```python
from build123d import *
from build123d.topology import SkipClean

# Parameters (mm, degrees)
EXTRUDE_1_DEPTH          = 2.75
SKETCH_2_R               = 9.5
CUT_EXTRUDE_1_DEPTH      = 87.748932825
SKETCH_3_R               = 1.65
CUT_EXTRUDE_2_DEPTH      = 87.748932825
CUT_EXTRUDE_3_DEPTH      = 87.748932825
CUT_EXTRUDE_3_DEPTH_BACK = 87.748932825
SKETCH_4_R               = 13
PATTERN_CIRCULAR_1_COUNT = 4
SKETCH_6_R               = 1.6
CUT_EXTRUDE_5_DEPTH      = 87.748932825
CUT_EXTRUDE_4_DEPTH      = 87.748932825
CUT_EXTRUDE_4_DEPTH_BACK = 87.748932825
SKETCH_5_R               = 15
CUT_EXTRUDE_7_DEPTH      = 87.748932825
CUT_EXTRUDE_7_DEPTH_BACK = 87.748932825
SKETCH_8_R               = 1.6


with BuildPart() as part:
    # ｽｹｯﾁ1 → ﾎﾞｽ - 押し出し1 (new, symmetric)
    with BuildSketch(Plane.XY):
        with BuildLine():
            Line((17.5, 0), (-47.316776584, 0))
            Line((-47.316776584, 0), (-47.316776584, -50))
            ThreePointArc((-47.316776584, -50), (-28.966828956, -72.113956347), (-3.847704112, -58.157695734))
            Line((-3.847704112, -58.157695734), (16.309278589, -6.34487446))
            ThreePointArc((16.309278589, -6.34487446), (17.199743825, -3.227818512), (17.5, 0))
        make_face()
    extrude_1 = extrude(amount=EXTRUDE_1_DEPTH, both=True)

    # ｽｹｯﾁ2 → ｶｯﾄ - 押し出し1 (cut, symmetric)
    with BuildSketch(Plane.XY.offset(2.75)):
        Circle(SKETCH_2_R)
    cut_extrude_1 = extrude(amount=CUT_EXTRUDE_1_DEPTH, both=True, mode=Mode.SUBTRACT)

    # ｽｹｯﾁ3 → ｶｯﾄ - 押し出し2 (cut, symmetric)
    with BuildSketch(Plane.XY.offset(2.75)):
        with Locations((-24.816776584, -67.5)):
            Circle(SKETCH_3_R)
    cut_extrude_2 = extrude(amount=CUT_EXTRUDE_2_DEPTH, both=True, mode=Mode.SUBTRACT)

    # ｽｹｯﾁ4 → ｶｯﾄ - 押し出し3 (cut, two sides: drawn at the far end of the back side and taken through both)
    with BuildSketch(Plane.XY.offset(2.75).offset(-CUT_EXTRUDE_3_DEPTH_BACK)):
        with Locations((-24.816776584, -50)):
            Circle(SKETCH_4_R)
    extrude(amount=CUT_EXTRUDE_3_DEPTH + CUT_EXTRUDE_3_DEPTH_BACK, mode=Mode.SUBTRACT)

    # 円形ﾊﾟﾀｰﾝ1: ｶｯﾄ - 押し出し2 ×4 about axis
    pattern_circular_1_axis = Axis((-24.816776584, -50, 0), (0, 0, 1))
    for i in range(1, PATTERN_CIRCULAR_1_COUNT):
        add(cut_extrude_2.rotate(pattern_circular_1_axis, i * 360 / PATTERN_CIRCULAR_1_COUNT), mode=Mode.SUBTRACT)

    # ｽｹｯﾁ6 → ｶｯﾄ - 押し出し5 (cut, through all)
    with BuildSketch(Plane.XY.offset(2.75)):
        with Locations((-2, -37)):
            Circle(SKETCH_6_R)
    cut_extrude_5 = extrude(amount=-CUT_EXTRUDE_5_DEPTH, mode=Mode.SUBTRACT)

    # ﾐﾗｰ1: ﾎﾞｽ - 押し出し1, ｶｯﾄ - 押し出し1, ｶｯﾄ - 押し出し5 across plane
    with SkipClean():  # the faces are left unmerged after this step: merging them gives an invalid solid
        add(extrude_1.mirror(Plane.ZX))
        add(cut_extrude_1.mirror(Plane.ZX), mode=Mode.SUBTRACT)
        add(cut_extrude_5.mirror(Plane.ZX), mode=Mode.SUBTRACT)

    # ｽｹｯﾁ5 → ｶｯﾄ - 押し出し4 (cut, two sides: drawn at the far end of the back side and taken through both)
    with SkipClean():  # the faces are left unmerged after this step: merging them gives an invalid solid
        with BuildSketch(Plane.XY.offset(2.75).offset(-CUT_EXTRUDE_4_DEPTH_BACK)):
            with Locations((-24.816776584, 50)):
                Circle(SKETCH_5_R)
        extrude(amount=CUT_EXTRUDE_4_DEPTH + CUT_EXTRUDE_4_DEPTH_BACK, mode=Mode.SUBTRACT)

    # ｽｹｯﾁ8 → ｶｯﾄ - 押し出し7 (cut, two sides: drawn at the far end of the back side and taken through both)
    with SkipClean():  # the faces are left unmerged after this step: merging them gives an invalid solid
        with BuildSketch(Plane.XY.offset(2.75).offset(-CUT_EXTRUDE_7_DEPTH_BACK)):
            with Locations((-42.316776584, 15)):
                Circle(SKETCH_8_R)
            with Locations((-42.316776584, -15)):
                Circle(SKETCH_8_R)
        extrude(amount=CUT_EXTRUDE_7_DEPTH + CUT_EXTRUDE_7_DEPTH_BACK, mode=Mode.SUBTRACT)


solid = part.part
```
Source: CAD feature listing. Evaluate the final solid. Frame: model axes, mm. Round coordinates to 2 decimals unless told otherwise and drop trailing zeros. Write each loop counter-clockwise with the first axis right and the second up, starting at its lowest first coordinate (ties: lowest second). Pieces come first, ordered by that corner, then holes. Notation, with made-up numbers: M 67.5,-31 L 114.5,-31 A11 ccw 114.5,-25 Z; hole C 8,40 d8. An arc over 180 degrees is marked long. Answer as a JSON object with one key per item and string values. Group by question number.
(1) Mould query, pull axis X, two halves, no side actions, for faces 1 (the flat face through (-23, 1, 2.75)), 2 (the cylindrical face through (-29.39, 72.03, 0.04)), 3 (the cylindrical face through (-1.26, -38.42, 0.04)), 4 (the cylindrical face through (-24.602, -34.136, 0.038)). Classes: +X half, -X half, draft (parallel to the pull), parting line (faces both ways), or undercut.
(2) Section query C-C on x = -2. Output: boundary loops of the cut face in (y, z).
(3) Section query B-B on y = 37. Output: boundary loops of the cut face in (x, z).
(4) Section query D-D on y = 1.5. Output: boundary loops of the cut face in (x, z), then the cut area to 3 significant figures.
(5) Section query A-A on x = -35.5. Output: boundary loops of the cut face in (y, z), then the cut area to 3 significant figures.
(6) Ray query, line 1 (Y direction, x = -41, z = -1.55); line 2 (X direction, y = -50, z = -0.55); line 3 (Y direction, x = -31, z = 0.6). Return the intervals inside material, ascending. Write a range as [from, to].
(7) First-contact query: pin 1 (1.5 mm diameter, centred on y = -9.5, z = 1, fed in from +X). Flat tip, straight axial feed; report the tip coordinate or a pass-through.
Computed values:
{
 "1": {"face 1": "draft", "face 2": "parting line", "face 3": "undercut", "face 4": "undercut"},
 "2": {"outline": "M -53.41,-2.75 L -38.6,-2.75 L -38.6,2.75 L -53.41,2.75 Z; M -35.4,-2.75 L -9.29,-2.75 L -9.29,2.75 L -35.4,2.75 Z; M 9.29,-2.75 L 35.4,-2.75 L 35.4,2.75 L 9.29,2.75 Z; M 38.6,-2.75 L 53.41,-2.75 L 53.41,2.75 L 38.6,2.75 Z"},
 "3": {"outline": "M -47.32,-2.75 L -32.3,-2.75 L -32.3,2.75 L -47.32,2.75 Z; M -17.33,-2.75 L -3.6,-2.75 L -3.6,2.75 L -17.33,2.75 Z; M -0.4,-2.75 L 4.38,-2.75 L 4.38,2.75 L -0.4,2.75 Z"},
 "4": {"outline": "M -47.32,-2.75 L -9.38,-2.75 L -9.38,2.75 L -47.32,2.75 Z; M 9.38,-2.75 L 17.44,-2.75 L 17.44,2.75 L 9.38,2.75 Z", "area": "253 mm^2"},
 "5": {"outline": "M -69.8,-2.75 L -57.41,-2.75 L -57.41,2.75 L -69.8,2.75 Z; M -42.59,-2.75 L 39.47,-2.75 L 39.47,2.75 L -42.59,2.75 Z; M 60.53,-2.75 L 69.8,-2.75 L 69.8,2.75 L 60.53,2.75 Z", "area": "571 mm^2"},
 "6": {"line 1": "[-65.63, -50.99], [-49.01, -15.91], [-14.09, 14.09], [15.91, 65.63]", "line 2": "[-47.32, -43.97], [-40.67, -37.82], [-11.82, -8.97], [-5.67, -0.67]", "line 3": "[-71.63, -61.44], [-38.56, 36.33], [63.67, 71.63]"},
 "7": {"pin 1": "x = 15.37"}
}
